Verification items for the finished model (mm, model axes). Give positions to 0.01 mm unless a question says otherwise; leave off trailing zeros. Loops run counter-clockwise (first coordinate to the right, second up) from the corner with the lowest first, then second, coordinate; pieces in that order, holes last. Notation, with made-up numbers: M 27.25,68 L 35.25,68 A38 ccw 35.25,106 Z; hole C 20,-39 d6. An arc over 180 degrees is marked long. Use a Markdown table: item, result.
from build123d import *

# Parameters (mm, degrees)
SKETCH1_W                = 120
SKETCH1_H                = 110
BOSS_EXTRUDE1_DEPTH      = 18
F_5_0_5_DIAMETER_HOLE1_D = 5
F_5_0_5_DIAMETER_HOLE3_D = 5


with BuildPart() as part:
    # Sketch1 → Boss-Extrude1 (new body)
    with BuildSketch(Plane(origin=(0, 0, 0), x_dir=(1, 0, 0), z_dir=(0, 1, 0))):
        Rectangle(SKETCH1_W, SKETCH1_H)
    extrude(amount=BOSS_EXTRUDE1_DEPTH)

    # Ø5.0 (5) Diameter Hole1 (through all)
    with Locations(Plane(origin=(0, 0, 0), x_dir=(-1, 0, 0), z_dir=(0, -1, 0))):
        with Locations((-20, 46), (35, 46), (35, -46), (-20, -46)):
            Hole(F_5_0_5_DIAMETER_HOLE1_D / 2)

    # Ø5.0 (5) Diameter Hole3 (through all)
    with Locations(Plane(origin=(0, 0, 0), x_dir=(-1, 0, 0), z_dir=(0, -1, 0))):
        with Locations((8, 20), (-30, 20), (-30, -20), (8, -20)):
            Hole(F_5_0_5_DIAMETER_HOLE3_D / 2)


solid = part.part
(1) Cross-section at B-B on x = 20. Record the cut outline in (y, z), then the cut area to 3 significant figures.
Results below:
| item | result |
|---|---|
| outline | M 0,-55 L 18,-55 L 18,-48.5 L 0,-48.5 Z; M 0,-43.5 L 18,-43.5 L 18,43.5 L 0,43.5 Z; M 0,48.5 L 18,48.5 L 18,55 L 0,55 Z |
| area | 1,800 mm^2 |
(2) Material ranges on line 1 (X direction, y = 14, z = 46); line 2 (X direction, y = 11.5, z = 20); line 3 (Z direction, x = 30, y = 13.5), recorded low to high.
Results below:
| item | result |
|---|---|
| line 1 | -60 to -37.5, -32.5 to 17.5, 22.5 to 60 |
| line 2 | -60 to -10.5, -5.5 to 27.5, 32.5 to 60 |
| line 3 | -55 to -22.5, -17.5 to 17.5, 22.5 to 55 |
(3) Draft check along Z on faces 1 (the cylindrical face through (28.16, 9.13, 18.31)), 2 (the cylindrical face through (-32.69, 9.13, 46.96)), 3 (the flat face through (-1, 9, 55)), 4 (the flat face through (-60, 9, 1)). Enter one of: +Z half, -Z half, draft (parallel to the pull), parting line (faces both ways), or undercut.
Results below:
| item | result |
|---|---|
| face 1 | undercut |
| face 2 | undercut |
| face 3 | +Z half |
| face 4 | draft |
(4) Cross-section at A-A on z = -20. Record the cut outline in (x, y).
Results below:
| item | result |
|---|---|
| outline | M -60,0 L -10.5,0 L -10.5,18 L -60,18 Z; M -5.5,0 L 27.5,0 L 27.5,18 L -5.5,18 Z; M 32.5,0 L 60,0 L 60,18 L 32.5,18 Z |
